from build123d import *

# Parameters (mm, degrees)
BOSS_EXTRUDE1_DEPTH = 37.465
SKETCH3_R           = 7.332348419
SKETCH3_R_2         = 6.875
SKETCH3_R_3         = 2.5527
CUT_EXTRUDE1_DEPTH  = 76.555216453


with BuildPart() as part:
    # Sketch1 → Boss-Extrude1 (new, symmetric)
    with BuildSketch(Plane(origin=(0, 0, 0), x_dir=(0, 0, -1), z_dir=(1, 0, 0))):
        Polygon((7.332348419, 0), (3.666174209, 6.35), (-3.666174209, 6.35), (-7.332348419, 0), (-3.666174209, -6.35), (3.666174209, -6.35), align=None)
    extrude(amount=BOSS_EXTRUDE1_DEPTH, both=True)

    # Sketch2 → Cut-Revolve1 (revolve, cut)
    with BuildSketch(Plane(origin=(0, 0, 0), x_dir=(1, 0, 0), z_dir=(0, 1, 0))):
        Polygon((34.925, -5.8547), (35.9156, -5.8547), (35.9156, -6.35), (37.465, -6.35), (37.465, -8.89), (34.925, -8.89), align=None)
    cut_revolve1 = revolve(axis=Axis((0, 0, 0), (1, 0, 0)), mode=Mode.SUBTRACT)

    # Mirror1: Cut-Revolve1 across plane
    add(cut_revolve1.mirror(Plane(origin=(0, 0, 0), x_dir=(0, 0, 1), z_dir=(1, 0, 0))), mode=Mode.SUBTRACT)

    # Sketch3 → Cut-Extrude1 (cut, through all)
    # profile 1 of 2: a face of its own
    with BuildSketch(Plane(origin=(37.465, 0, 0), x_dir=(0, 0, -1), z_dir=(1, 0, 0))):
        Circle(SKETCH3_R)
        Circle(SKETCH3_R_2, mode=Mode.SUBTRACT)
    # profile 2 of 2: a face of its own
    with BuildSketch(Plane(origin=(37.465, 0, 0), x_dir=(0, 0, -1), z_dir=(1, 0, 0))):
        Circle(SKETCH3_R_3)
    extrude(amount=-CUT_EXTRUDE1_DEPTH, mode=Mode.SUBTRACT)


solid = part.part
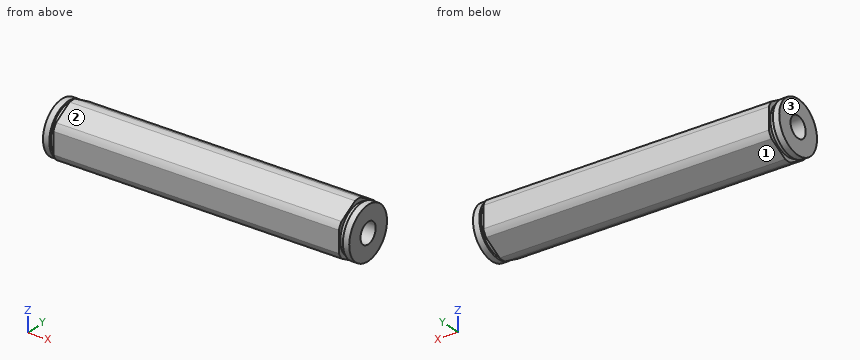
CAD build for the part. Positions are in the model's coordinates, mm. Face numbers are marked on the shaded views. Give positions to 0.01 mm unless a question says otherwise; leave off trailing zeros. Order: outer loops, then holes, each group sorted by start corner. A loop starts at its lowest first (then second) coordinate and runs counter-clockwise, first axis right, second up. Notation, with made-up numbers: (59.25, 9.25) -> (64.25, 9.25) arc R18 ccw to (64.25, 23.25) -> close; hole circle Ø2 at (37.25, 25.5). An arc over 180 degrees is marked (long way). Return JSON: item names as keys, results as strings.
Q1. Saw through at B-B (y = 0). Write the cut outline in (x, z) (3 decimals).
Working result:
{"outline": "(-37.465, -6.35) -> (-35.916, -6.35) -> (-35.916, -5.855) -> (-34.925, -5.855) -> (-34.925, -6.875) -> (34.925, -6.875) -> (34.925, -5.855) -> (35.916, -5.855) -> (35.916, -6.35) -> (37.465, -6.35) -> (37.465, -2.553) -> (-37.465, -2.553) -> close; (-37.465, 2.553) -> (37.465, 2.553) -> (37.465, 6.35) -> (35.916, 6.35) -> (35.916, 5.855) -> (34.925, 5.855) -> (34.925, 6.875) -> (-34.925, 6.875) -> (-34.925, 5.855) -> (-35.916, 5.855) -> (-35.916, 6.35) -> (-37.465, 6.35) -> close"}
Q2. Drill centre lines: line 1 (X direction, y = 0, z = -6) (3 decimals); line 2 (Y direction, x = 1, z = 0); line 3 (Z direction, x = 34.5, y = 2). Where is each one in solid material? Low to high.
Working result:
{"line 1": "-37.465 to -35.916, -34.925 to 34.925, 35.916 to 37.465", "line 2": "-6.35 to -2.55, 2.55 to 6.35", "line 3": "-6.18 to -1.59, 1.59 to 6.18"}
Q3. Saw through at C-C (z = 0). Write the cut outline in (x, y) (3 decimals), then the cut area to 3 significant figures.
Working result:
{"outline": "(-37.465, -6.35) -> (-35.916, -6.35) -> (-35.916, -5.855) -> (-34.925, -5.855) -> (-34.925, -6.35) -> (34.925, -6.35) -> (34.925, -5.855) -> (35.916, -5.855) -> (35.916, -6.35) -> (37.465, -6.35) -> (37.465, -2.553) -> (-37.465, -2.553) -> close; (-37.465, 2.553) -> (37.465, 2.553) -> (37.465, 6.35) -> (35.916, 6.35) -> (35.916, 5.855) -> (34.925, 5.855) -> (34.925, 6.35) -> (-34.925, 6.35) -> (-34.925, 5.855) -> (-35.916, 5.855) -> (-35.916, 6.35) -> (-37.465, 6.35) -> close", "area": "567 mm²"}
Q4. Flat gauge pins, fed straight in: pin 1 (1 mm diameter, centred on x = -27.5, y = 1.5, fed in from -Z) (3 decimals); pin 2 (4 mm diameter, centred on x = 27, y = -2.5, fed in from -Z); pin 3 (6.5 mm diameter, centred on y = 2, z = -1.5, fed in from -X) (3 decimals). Where does each tip first touch, or does it go through?
Working result:
{"pin 1": "z = -6.755", "pin 2": "z = -6.86", "pin 3": "x = -37.465"}
Q5. Saw through at A-A (x = 30.5). Write the cut outline in (y, z) (3 decimals).
Working result:
{"outline": "(-6.35, -2.635) arc R6.875 ccw to (-5.457, -4.182) -> (-0.893, -6.817) arc R6.875 ccw to (0.893, -6.817) -> (5.457, -4.182) arc R6.875 ccw to (6.35, -2.635) -> (6.35, 2.635) arc R6.875 ccw to (5.457, 4.182) -> (0.893, 6.817) arc R6.875 ccw to (-0.893, 6.817) -> (-5.457, 4.182) arc R6.875 ccw to (-6.35, 2.635) -> close; hole circle Ø5.105 at (0, 0)"}
Q6. Mould opens along Y. For the marked faces 1, 2 and 3 say: pulls with the +Y half, pulls with the -Y half, needs draft (parallel to the pull), parting line crosses it, or undercut.
Working result:
{"face 1": "pulls with the +Y half", "face 2": "pulls with the -Y half", "face 3": "needs draft"}
